```python
from build123d import *

# Parameters (mm, degrees)
F0_R     = 33
F1_DEPTH = 3.2
F2_R     = 9
F3_DEPTH = 6.401
F4_SIZE2 = 5.459553514
F4_SIZE  = 15


with BuildPart() as f1:
    # F0 (on Top) → F1 (new body, symmetric)
    with BuildSketch(Plane.XY):
        Circle(F0_R)
    extrude(amount=F1_DEPTH, both=True)

    # F2 (on face) → F3 (cut, through all)
    with BuildSketch(Plane.XY.offset(3.2)):
        Circle(F2_R)
    extrude(amount=-F3_DEPTH, mode=Mode.SUBTRACT)

    # F4
    f4_edges = [f1.edges().sort_by_distance(p)[0] for p in [
        (-33, 0, 3.2),
    ]]
    f4_side = f1.faces().sort_by_distance((-32.066619, 0, 3.2))[0]
    chamfer(f4_edges, length=F4_SIZE, length2=F4_SIZE2, reference=f4_side)


solid = f1.part
```
Geometry: final body of the model. Coordinates: model frame, mm. Round coordinates to 2 decimals unless told otherwise and drop trailing zeros. Order: outer loops, then holes, each group sorted by start corner. A loop starts at its lowest first (then second) coordinate and runs counter-clockwise, first axis right, second up. Notation, with made-up numbers: (17.25, 3) - (76.25, 3) arc R8 cw to (76.25, 15) - close; hole circle Ø6 at (59.5, -30.75). An arc over 180 degrees is marked (long way). Use CSV: the item, a comma, the result in double quotes. Start each with the question number.
Q1. Section query C-C (z = 1.25). Return loops of the section in (x, y).
Q2. First-contact query: pin 1 (4 mm diameter, centred on x = -24.5, y = -11, fed in from +Z). Flat tip, straight axial feed; report the tip coordinate or a pass-through.
Q3. Material intervals for line 1 along Z through (x, y) = (19, -17); line 2 along Z through (x, y) = (23.5, 12.5); line 3 along Y through (x, z) = (-13.5, -3), sorted ascending. Write a range as from..to.
Q4. Section query A-A (x = 0). Return loops of the section in (y, z).
Q5. Mould query, pull axis X, two halves, no side actions, for faces 1 (the face through (-1.172, 8.923, 0.045)), 2 (the face through (30.5, -12.6, -2.7)), 3 (the face through (-8.3, 4.3, 3.2)). Classes: +X half, -X half, draft (parallel to the pull), parting line (faces both ways), or undercut.
Result set:
1,outline,"circle Ø46.72 at (0, 0); hole circle Ø18 at (0, 0)"
2,pin 1,"stops at z = 0.7"
3,line 1,"z = -3.2..0.47"
3,line 2,"z = -3.2..0.06"
3,line 3,"y = -30.11..30.11"
4,outline,"(-33, -3.2) - (-9, -3.2) - (-9, 3.2) - (-18, 3.2) - (-33, -2.26) - close; (9, -3.2) - (33, -3.2) - (33, -2.26) - (18, 3.2) - (9, 3.2) - close"
5,face 1,"undercut"
5,face 2,"parting line"
5,face 3,"draft"
